Check sheet for the drawn part. Datum: minimum x, y, z corner. Units: mm. A direction names the side the tool comes from. Round coordinates to 2 decimals unless told otherwise and drop trailing zeros. Order: outer loops, then holes, each group sorted by start corner. A loop starts at its lowest first (then second) coordinate and runs counter-clockwise, first axis right, second up. Notation, with made-up numbers: (-29.75, 86.5) -> (16.25, 86.5) arc R18 ccw to (16.25, 110.5) -> close; hole circle Ø9 at (-7.5, 35). An arc over 180 degrees is marked (long way). Answer as CSV lines item,"result". Start each with the question number.
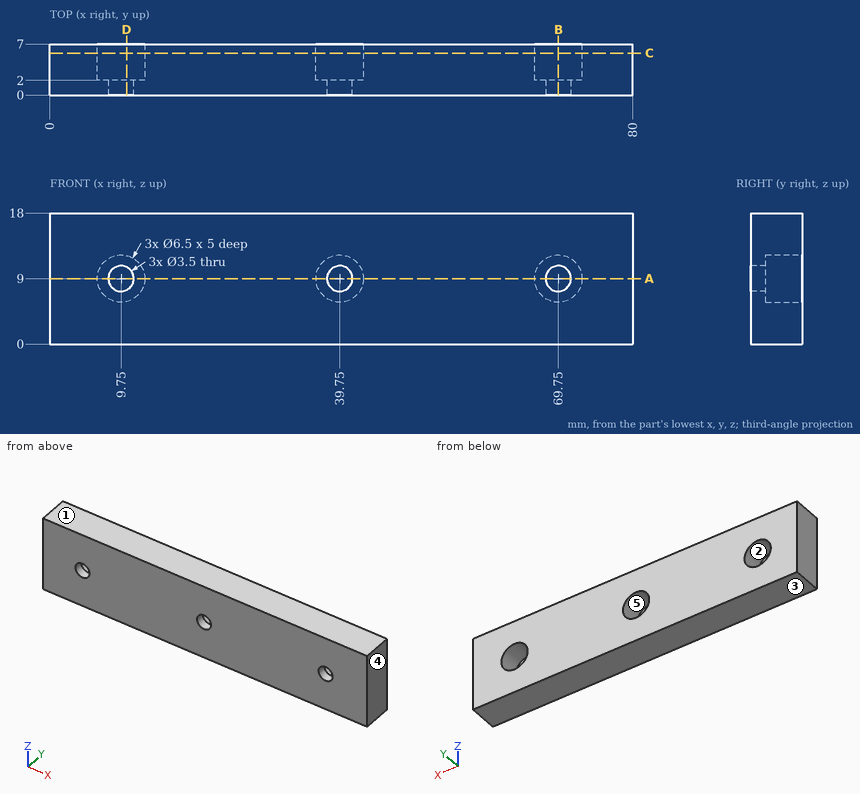
1) Mould release check, pull along Z, two halves, no side actions. Record for the marked faces 1, 2 and 3: released by +Z, released by -Z, zero draft, split by the parting line, or undercut.
2) Section check A-A on z = 9. Record the cut outline in (x, y), then the cut area to 4 significant figures.
3) Section check B-B on x = 69.75. Record the cut outline in (y, z).
4) Section check C-C on y = 5.75. Record the cut outline in (x, z).
5) Access from +Z, -Z, +X, -X, +Y, -Y to the whole of each face (thin tool, end or side, straight path). Record for the marked faces 4 and 5.
6) Material ranges on line 1 along X through (y, z) = (3.3, 9); line 2 along Z through (x, y) = (9.75, 1.3); line 3 along X through (y, z) = (1, 8.25), recorded low to high.
7) Section check D-D on x = 10.5. Record the cut outline in (y, z), then the cut area to 3 significant figures.
8) Depth check by flat-ended pin: pin 1 Ø2 at (x, z) = (39.75, 9) entering from -Y; pin 2 Ø4 at (x, z) = (9.75, 9) entering from +Y. Enter the tip coordinate at first touch or a pass-through.
Solutions:
1,face 1,"released by +Z"
1,face 2,"undercut"
1,face 3,"released by -Z"
2,outline,"(0, 0) -> (8, 0) -> (8, 2) -> (6.5, 2) -> (6.5, 7) -> (0, 7) -> close; (11.5, 0) -> (38, 0) -> (38, 2) -> (36.5, 2) -> (36.5, 7) -> (13, 7) -> (13, 2) -> (11.5, 2) -> close; (41.5, 0) -> (68, 0) -> (68, 2) -> (66.5, 2) -> (66.5, 7) -> (43, 7) -> (43, 2) -> (41.5, 2) -> close; (71.5, 0) -> (80, 0) -> (80, 7) -> (73, 7) -> (73, 2) -> (71.5, 2) -> close"
2,area,"441.5 mm^2"
3,outline,"(0, 0) -> (7, 0) -> (7, 5.75) -> (2, 5.75) -> (2, 7.25) -> (0, 7.25) -> close; (0, 10.75) -> (2, 10.75) -> (2, 12.25) -> (7, 12.25) -> (7, 18) -> (0, 18) -> close"
4,outline,"(0, 0) -> (80, 0) -> (80, 18) -> (0, 18) -> close; hole circle Ø6.5 at (9.75, 9); hole circle Ø6.5 at (39.75, 9); hole circle Ø6.5 at (69.75, 9)"
5,face 4,"+Z, -Z, +X, +Y, -Y"
5,face 5,"+Y"
6,line 1,"x = 0 to 6.5, 13 to 36.5, 43 to 66.5, 73 to 80"
6,line 2,"z = 0 to 7.25, 10.75 to 18"
6,line 3,"x = 0 to 8.17, 11.33 to 38.17, 41.33 to 68.17, 71.33 to 80"
7,outline,"(0, 0) -> (7, 0) -> (7, 5.84) -> (2, 5.84) -> (2, 7.42) -> (0, 7.42) -> close; (0, 10.58) -> (2, 10.58) -> (2, 12.16) -> (7, 12.16) -> (7, 18) -> (0, 18) -> close"
7,area,"88.1 mm^2"
8,pin 1,"passes through"
8,pin 2,"stops at y = 2"
